The drawing under review shows one solid part. Ordinate dimensions are in mm from its lowest x, y, z. A direction names the side the tool comes from. Coordinates: 2 decimals unless noted, no trailing zeros. Loops run counter-clockwise (first coordinate to the right, second up) from the corner with the lowest first, then second, coordinate; pieces in that order, holes last. Notation, with made-up numbers: M -36,-0.5 L -31,-0.5 A19 ccw -31,31.5 Z; hole C -1,58 d2. An arc over 180 degrees is marked long. Answer as a JSON object with one key per item and string values. Group by question number.
1. Insertion check: pin 1 (15 mm diameter, centred on y = 65, z = 72.5, fed in from -X); pin 2 (2 mm diameter, centred on y = 60.5, z = 51.5, fed in from +X); pin 3 (0.8 mm diameter, centred on x = 1.5, z = 47, fed in from +Y). Each pin has a flat end and moves straight along its axis. Give the tip position at first contact, or say it passes through.
2. To check wall thickness, follow probe 1 along Y at (x, z) = (3.45, 50); probe 2 along Z at (x, y) = (3.85, 62.5); probe 3 along X at (y, z) = (69, 71). State the ranges of each line that lie inside material, in increasing order.
3. Consider section A-A (y = 62.5). State the section outline as (x, z) points.
4. Machinability: for the marked faces 1 and 2, which of the approach directions +Z, -Z, +X, -X, +Y, -Y give a long, thin tool a straight path to every point of the face, cutting with its end or side? Answer none if there is none.
5. Consider section B-B (z = 26). State the section outline as (x, y) points, then the cut area to 3 significant figures.
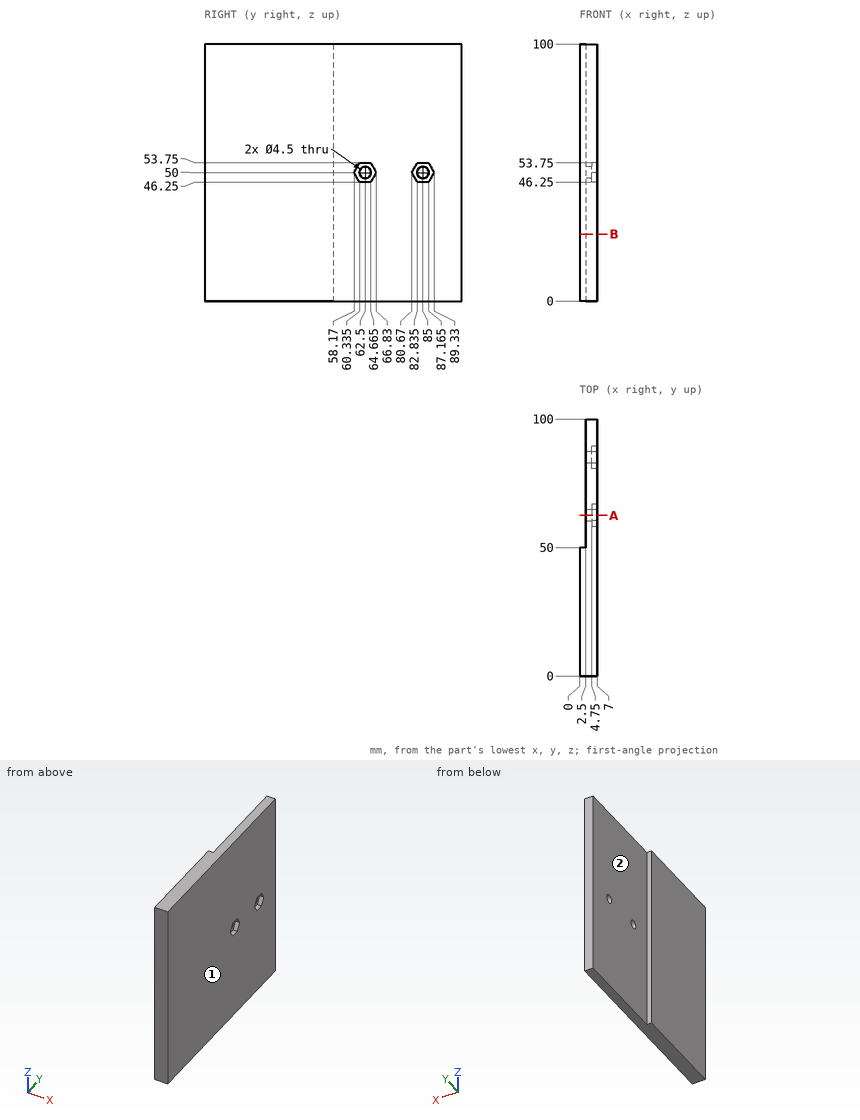
Findings below:
{
 "1": {"pin 1": "stops at x = 2.5", "pin 2": "stops at x = 4.75", "pin 3": "stops at y = 50"},
 "2": {"probe 1": "y = 0 to 60.25, 64.75 to 82.75, 87.25 to 100", "probe 2": "z = 0 to 47.75, 52.25 to 100", "probe 3": "x = 2.5 to 7"},
 "3": {"outline": "M 2.5,0 L 7,0 L 7,46.25 L 4.75,46.25 L 4.75,47.75 L 2.5,47.75 Z; M 2.5,52.25 L 4.75,52.25 L 4.75,53.75 L 7,53.75 L 7,100 L 2.5,100 Z"},
 "4": {"face 1": "+Z, -Z, +X, +Y, -Y", "face 2": "+Z, -Z, -X, +Y"},
 "5": {"outline": "M 0,0 L 7,0 L 7,100 L 2.5,100 L 2.5,50 L 0,50 Z", "area": "575 mm^2"}
}
